Could you check a few things on this model? Use its own coordinates, in mm. Round coordinates to 2 decimals unless told otherwise and drop trailing zeros. Write each loop counter-clockwise with the first axis right and the second up, starting at its lowest first coordinate (ties: lowest second). Pieces come first, ordered by that corner, then holes. Notation, with made-up numbers: (35.5, 55.5) -> (88.5, 55.5) arc R27 cw to (88.5, 74.5) -> close; hole circle Ø2 at (87.25, 84.25). An arc over 180 degrees is marked (long way). Return JSON: item names as keys, results as strings.
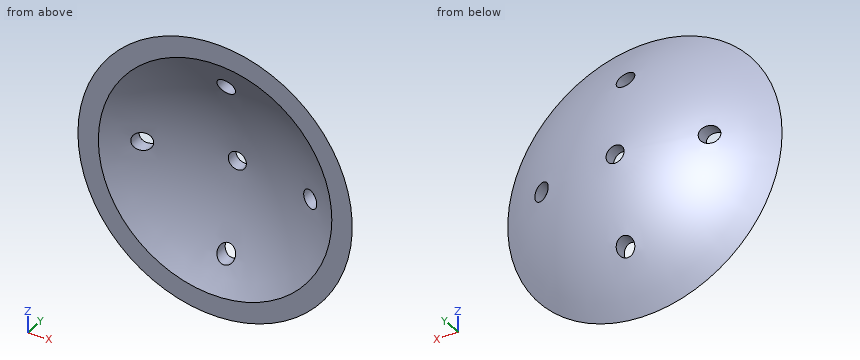
from build123d import *

# Parameters (mm, degrees)
SKETCH3_W          = 96.508277199
SKETCH3_H          = 68.977702825
CUT_EXTRUDE1_DEPTH = 100
SKETCH5_R          = 1.5
CUT_EXTRUDE2_DEPTH = 100
SKETCH6_R          = 1.5
CUT_EXTRUDE3_DEPTH = 100


with BuildPart() as part:
    # Sketch1 → Revolve1 (revolve)
    with BuildSketch(Plane.XY):
        with BuildLine():
            Line((0, 37), (0, 0))
            Line((0, 0), (0, -37))
            ThreePointArc((0, -37), (-37, 0), (0, 37))
        make_face()
    revolve(axis=Axis((0, 51.787709497, 0), (0, -1, 0)))

    # Sketch3 → Cut-Extrude1 (cut, symmetric)
    with BuildSketch(Plane.XY):
        with Locations((2.168158787, -5.395185821)):
            Rectangle(SKETCH3_W, SKETCH3_H)
    extrude(amount=CUT_EXTRUDE1_DEPTH, both=True, mode=Mode.SUBTRACT)

    # Sketch4 → Cut-Revolve1 (revolve, cut)
    with BuildSketch(Plane.XY):
        with BuildLine():
            Line((0, 0), (0, 35))
            ThreePointArc((0, 35), (-35, 0), (0, -35))
            Line((0, -35), (0, 0))
        make_face()
    revolve(axis=Axis((0, 39.939026177, 0), (0, -1, 0)), mode=Mode.SUBTRACT)

    # Sketch5 → Cut-Extrude2 (cut, symmetric)
    with BuildSketch(Plane(origin=(0, 0, 0), x_dir=(1, 0, 0), z_dir=(0, 1, 0))):
        with Locations(Location((0, 14, 0), (0, 0, 122.347198926))):
            Circle(SKETCH5_R)
        with Locations((14, 0)):
            Circle(SKETCH5_R)
        with Locations(Location((0, -14, 0), (0, 0, 148.968284828))):
            Circle(SKETCH5_R)
        with Locations(Location((-14, 0, 0), (0, 0, 359.999999797))):
            Circle(SKETCH5_R)
    extrude(amount=CUT_EXTRUDE2_DEPTH, both=True, mode=Mode.SUBTRACT)

    # Sketch6 → Cut-Extrude3 (cut, symmetric)
    with BuildSketch(Plane(origin=(0, 0, 0), x_dir=(1, 0, 0), z_dir=(0, 1, 0))):
        with Locations(Location((0, 0, 0), (0, 0, 90))):
            Circle(SKETCH6_R)
    extrude(amount=CUT_EXTRUDE3_DEPTH, both=True, mode=Mode.SUBTRACT)


solid = part.part
1) I want a section at C-C, the plane x = -14. Please give me the cut outline in (y, z), and give its area (3 significant figures).
Return value:
{"outline": "(29.09, -18.07) arc R34.25 ccw to (34.22, -1.5) -> (32.04, -1.5) arc R32.08 cw to (29.09, -13.51) -> close; (29.09, 13.51) arc R32.08 cw to (32.04, 1.5) -> (34.22, 1.5) arc R34.25 ccw to (29.09, 18.07) -> close", "area": "65.4 mm²"}
2) I want a section at D-D, the plane y = 35.75. Please give me the cut outline in (x, z), and give its area (3 significant figures).
Return value:
{"outline": "circle Ø19.07 at (0, 0); hole circle Ø3 at (0, 0)", "area": "279 mm²"}
3) Will these pins go through, and if not, where does the flat tip stop? pin 1 Ø4 at (x, y) = (-18, 31.5) entering from -Z; pin 2 Ø5 at (x, z) = (8, -4) entering from -Y; pin 3 Ø6 at (x, z) = (17, -13.5) entering from +Y.
Return value:
{"pin 1": "z = -13.92", "pin 2": "y = 33.08", "pin 3": "y = 31.92"}
4) If I drill on probe 1 along X at (y, z) = (30.25, -1.5); probe 2 along X at (y, z) = (32.1, 0); probe 3 along Y at (x, z) = (-3, 13.5), over which ranges is the centre line in solid material (lowest first)? Write a range as [from, to].
Return value:
{"probe 1": "[-21.25, -17.54], [17.54, 21.25]", "probe 2": "[-18.4, -15.5], [15.5, 18.4]", "probe 3": "[32.15, 34.32]"}
5) I want a section at B-B, the plane z = 14. Please give me the cut outline in (x, y).
Return value:
{"outline": "(-18.07, 29.09) -> (-13.51, 29.09) arc R32.08 cw to (-1.5, 32.04) -> (-1.5, 34.22) arc R34.25 ccw to start; (1.5, 32.04) arc R32.08 cw to (13.51, 29.09) -> (18.07, 29.09) arc R34.25 ccw to (1.5, 34.22) -> close"}
6) I want a section at A-A, the plane x = 0. Please give me the cut outline in (y, z).
Return value:
{"outline": "(29.09, -22.86) arc R37 ccw to (33.6, -15.5) -> (31.38, -15.5) arc R35 cw to (29.09, -19.46) -> close; (29.09, 19.46) arc R35 cw to (31.38, 15.5) -> (33.6, 15.5) arc R37 ccw to (29.09, 22.86) -> close; (32.69, -12.5) -> (34.82, -12.5) arc R37 ccw to (36.97, -1.5) -> (34.97, -1.5) arc R35 cw to start; (32.69, 12.5) arc R35 cw to (34.97, 1.5) -> (36.97, 1.5) arc R37 ccw to (34.82, 12.5) -> close"}
